```python
from build123d import *

# Parameters (mm, degrees)
SKETCH1_W           = 200
SKETCH1_H           = 200
SKETCH1_W_2         = 20
SKETCH1_H_2         = 5
SKETCH1_W_3         = 5
SKETCH1_H_3         = 20
BOSS_EXTRUDE1_DEPTH = 5


with BuildPart() as part:
    # Sketch1 → Boss-Extrude1 (new body)
    with BuildSketch(Plane.XY):
        Rectangle(SKETCH1_W, SKETCH1_H)
        with Locations((-42.738744268, 72.5)):
            Rectangle(SKETCH1_W_2, SKETCH1_H_2, mode=Mode.SUBTRACT)
        with Locations((31.360897281, 72.5)):
            Rectangle(SKETCH1_W_2, SKETCH1_H_2, mode=Mode.SUBTRACT)
        Polygon((-75, 57.435704121), (-70.001007164, 57.335351613), (-70.001007164, 37.335351613), (-75, 37.435704121), align=None, mode=Mode.SUBTRACT)
        with Locations((-72.5, -3.109084485)):
            Rectangle(SKETCH1_W_3, SKETCH1_H_3, mode=Mode.SUBTRACT)
        with Locations((-72.5, -50.464153422)):
            Rectangle(SKETCH1_W_3, SKETCH1_H_3, mode=Mode.SUBTRACT)
        with Locations((31.360897281, -72.5)):
            Rectangle(SKETCH1_W_2, SKETCH1_H_2, mode=Mode.SUBTRACT)
        with Locations((-42.738744268, -72.5)):
            Rectangle(SKETCH1_W_2, SKETCH1_H_2, mode=Mode.SUBTRACT)
        with Locations((72.5, -50.464153422)):
            Rectangle(SKETCH1_W_3, SKETCH1_H_3, mode=Mode.SUBTRACT)
        with Locations((72.5, -3.109084485)):
            Rectangle(SKETCH1_W_3, SKETCH1_H_3, mode=Mode.SUBTRACT)
        Polygon((75, 37.435704121), (70.001007164, 37.335351613), (70.001007164, 57.335351613), (75, 57.435704121), align=None, mode=Mode.SUBTRACT)
    extrude(amount=BOSS_EXTRUDE1_DEPTH)


solid = part.part
```
The model under review builds one solid part; all positions refer to its coordinate system, in mm. A direction names the side the tool comes from. Round coordinates to 2 decimals unless told otherwise and drop trailing zeros. Order: outer loops, then holes, each group sorted by start corner. A loop starts at its lowest first (then second) coordinate and runs counter-clockwise, first axis right, second up. Notation, with made-up numbers: (27.5, 71.5) -> (45.5, 71.5) arc R29 ccw to (45.5, 104.5) -> close; hole circle Ø1 at (13.25, -37.75). An arc over 180 degrees is marked (long way). One line per item, written item: value. Start each with the question number.
Q1. Mouldability with a two-part tool opening along X and no side actions: class faces 3 (the face through (-43, -75, 2)), 4 (the face through (-32.739, -73, 2)), 5 (the face through (100, -1, 2)), 6 (the face through (-1, 1, 5)) as released by +X, released by -X, zero draft, split by the parting line, or undercut.
Q2. Machinability: for faces 1 (the face through (70, -3, 2)), 2 (the face through (-1, -100, 2)), which of the approach directions +Z, -Z, +X, -X, +Y, -Y give a long, thin tool a straight path to every point of the face, cutting with its end or side? Answer none if there is none.
Q3. Wall thickness on line 1 (Y direction, x = -35, z = 3.05); line 2 (X direction, y = -73, z = 1.25): over which ranges is each line inside the solid? List them lowest first.
Q4. Take a section at C-C (z = 1.4). Count the separate pieces of the cut face and the enclosed holes in it, and give its area (3 significant figures).
Q5. Take a section at A-A (y = 53). Write out the cut boundary in (x, z).
Reported:
1. face 3: undercut
1. face 4: undercut
1. face 5: released by +X
1. face 6: zero draft
2. face 1: +Z, -Z
2. face 2: +Z, -Z, +X, -X, -Y
3. line 1: y = -100 to -75, -70 to 70, 75 to 100
3. line 2: x = -100 to -52.74, -32.74 to 21.36, 41.36 to 100
4. separate pieces: 1
4. enclosed holes: 10
4. area: 39,000 mm2
5. outline: (-100, 0) -> (-75, 0) -> (-75, 5) -> (-100, 5) -> close; (-70, 0) -> (70, 0) -> (70, 5) -> (-70, 5) -> close; (75, 0) -> (100, 0) -> (100, 5) -> (75, 5) -> close
